The model under review builds one solid part; all positions refer to its coordinate system, in mm. A direction names the side the tool comes from. Round coordinates to 2 decimals unless told otherwise and drop trailing zeros. Write each loop counter-clockwise with the first axis right and the second up, starting at its lowest first coordinate (ties: lowest second). Pieces come first, ordered by that corner, then holes. Notation, with made-up numbers: (6.5, -39) - (44.5, -39) arc R33 cw to (44.5, -3) - close; hole circle Ø2 at (3, 59.5). An arc over 180 degrees is marked (long way). Return JSON: item names as keys, results as strings.
from build123d import *

# Parameters (mm, degrees)
SKETCH1_W                   = 224.46234
SKETCH1_H                   = 149.606
BOSS_EXTRUDE1_DEPTH         = 2.54
SKETCH2_W                   = 44.45
SKETCH2_H                   = 87.5411
CUT_EXTRUDE1_DEPTH          = 135.899132423
F_1_4_CLEARANCE_HOLE1_D     = 6.5278
F_1_4_CLEARANCE_HOLE1_DEPTH = 9.398
F_1_4_CLEARANCE_HOLE1_TIP   = 1.961148974
SKETCH6_W                   = 25.4
SKETCH6_H                   = 2.54
CUT_EXTRUDE2_DEPTH          = 135.899132423
LPATTERN1_COUNT             = 4
LPATTERN1_PITCH             = 50.8
SKETCH7_W                   = 2.54
SKETCH7_H                   = 21.59
CUT_EXTRUDE3_DEPTH          = 135.899132423
LPATTERN2_COUNT             = 3
LPATTERN2_PITCH             = 43.18
SKETCH8_R                   = 9.525
CUT_EXTRUDE4_DEPTH          = 135.899132423
SKETCH9_R                   = 15.875
SKETCH9_W                   = 44.7802
SKETCH9_H                   = 69.85
CUT_EXTRUDE5_DEPTH          = 135.899132423
FILLET2_R                   = 12.7
SKETCH25_W                  = 12.7
SKETCH25_H                  = 147.066
BOSS_EXTRUDE5_DEPTH         = 2.54
SKETCH16_W                  = 2.54
SKETCH16_H                  = 25.4
BOSS_EXTRUDE2_DEPTH         = 2.54
SKETCH23_W                  = 44.45
SKETCH23_H                  = 87.5411
BOSS_EXTRUDE3_DEPTH         = 2.54
SKETCH24_W                  = 33.3375
SKETCH24_H                  = 149.606
BOSS_EXTRUDE4_DEPTH         = 2.54
LPATTERN3_COUNT             = 3
LPATTERN3_PITCH             = 50.8
LPATTERN3_COUNT_DIR2        = 2
LPATTERN3_PITCH_DIR2        = 273.03984
SKETCH18_W                  = 275.57984
SKETCH18_H                  = 5.334
CUT_EXTRUDE7_DEPTH          = 169.417839014
M3_CLEARANCE_HOLE1_D        = 3.2
M3_CLEARANCE_HOLE1_DEPTH    = 9.398
M3_CLEARANCE_HOLE1_TIP      = 0.96137699
SKETCH27_W                  = 73.9775
SKETCH27_H                  = 58.7375
CUT_EXTRUDE9_DEPTH          = 2.54
CUT_EXTRUDE10_DEPTH         = 2.54
SKETCH29_W                  = 25.4
SKETCH29_H                  = 2.54
CUT_EXTRUDE11_DEPTH         = 166.946131435
LPATTERN4_COUNT             = 5
LPATTERN4_PITCH             = 50.8


with BuildPart() as part:
    # Sketch1 → Boss-Extrude1 (new body)
    with BuildSketch(Plane(origin=(0, 0, 0), x_dir=(0, 0, -1), z_dir=(1, 0, 0))):
        Rectangle(SKETCH1_W, SKETCH1_H)
    extrude(amount=BOSS_EXTRUDE1_DEPTH)

    # Sketch2 → Cut-Extrude1 (cut, through all)
    with BuildSketch(Plane(origin=(2.54, 0, 0), x_dir=(0, 0, -1), z_dir=(1, 0, 0))):
        with Locations((90.00617, 31.03245)):
            Rectangle(SKETCH2_W, SKETCH2_H)
    extrude(amount=-CUT_EXTRUDE1_DEPTH, mode=Mode.SUBTRACT)

    # 1/4 Clearance Hole1
    with Locations(Plane(origin=(2.54, 0, 0), x_dir=(0, 0, -1), z_dir=(1, 0, 0))):
        with Locations((-81.69783, -64.77), (-62.01283, -64.77), (102.09657, -64.77), (82.41157, -64.77)):
            Hole(F_1_4_CLEARANCE_HOLE1_D / 2, depth=F_1_4_CLEARANCE_HOLE1_DEPTH)
            with Locations((0, 0, -(F_1_4_CLEARANCE_HOLE1_DEPTH + F_1_4_CLEARANCE_HOLE1_TIP / 2))):  # 118° drill point
                Cone(0, F_1_4_CLEARANCE_HOLE1_D / 2, F_1_4_CLEARANCE_HOLE1_TIP, mode=Mode.SUBTRACT)

    # Sketch6 → Cut-Extrude2 (cut, through all)
    with BuildSketch(Plane(origin=(2.54, 0, 0), x_dir=(0, 0, -1), z_dir=(1, 0, 0))):
        with Locations((39.84117, 73.533)):
            Rectangle(SKETCH6_W, SKETCH6_H)
    cut_extrude2 = extrude(amount=-CUT_EXTRUDE2_DEPTH, mode=Mode.SUBTRACT)

    # LPattern1: Cut-Extrude2 ×4
    with Locations(*[(0, 0, i * LPATTERN1_PITCH) for i in range(1, LPATTERN1_COUNT)]):
        add(cut_extrude2, mode=Mode.SUBTRACT)

    # Sketch7 → Cut-Extrude3 (cut, through all)
    with BuildSketch(Plane(origin=(2.54, 0, 0), x_dir=(0, 0, -1), z_dir=(1, 0, 0))):
        with Locations((66.51117, 53.213)):
            Rectangle(SKETCH7_W, SKETCH7_H)
    cut_extrude3 = extrude(amount=-CUT_EXTRUDE3_DEPTH, mode=Mode.SUBTRACT)

    # LPattern2: Cut-Extrude3 ×3
    with Locations(*[(0, -i * LPATTERN2_PITCH, 0) for i in range(1, LPATTERN2_COUNT)]):
        add(cut_extrude3, mode=Mode.SUBTRACT)

    # Sketch8 → Cut-Extrude4 (cut, through all)
    with BuildSketch(Plane(origin=(2.54, 0, 0), x_dir=(0, 0, -1), z_dir=(1, 0, 0))):
        with Locations((92.22867, -39.7370046)):
            Circle(SKETCH8_R)
        with Locations((-71.82993, -39.7370046)):
            Circle(SKETCH8_R)
    extrude(amount=-CUT_EXTRUDE4_DEPTH, mode=Mode.SUBTRACT)

    # Sketch9 → Cut-Extrude5 (cut, through all)
    with BuildSketch(Plane(origin=(2.54, 0, 0), x_dir=(0, 0, -1), z_dir=(1, 0, 0))):
        with Locations((-67.78625, 31.7373)):
            Circle(SKETCH9_R)
        with Locations((3.84937, -39.878)):
            Rectangle(SKETCH9_W, SKETCH9_H)
    extrude(amount=-CUT_EXTRUDE5_DEPTH, mode=Mode.SUBTRACT)

    # Fillet2
    fillet2_edges = [part.edges().sort_by_distance(p)[0] for p in [
        (1.27, -74.803, 18.54073),
        (1.27, -4.953, 18.54073),
        (1.27, -4.953, -26.23947),
        (1.27, -74.803, -26.23947),
    ]]
    fillet(fillet2_edges, radius=FILLET2_R)

    # Sketch25 → Boss-Extrude5 (add)
    with BuildSketch(Plane(origin=(2.54, 0, 0), x_dir=(0, 0, -1), z_dir=(1, 0, 0))):
        with Locations((-118.58117, -1.27)):
            Rectangle(SKETCH25_W, SKETCH25_H)
    extrude(amount=-BOSS_EXTRUDE5_DEPTH)

    # Sketch16 → Boss-Extrude2 (add)
    with BuildSketch(Plane(origin=(2.54, 0, 0), x_dir=(0, 0, -1), z_dir=(1, 0, 0))):
        with Locations((-126.20117, 34.163)):
            Rectangle(SKETCH16_W, SKETCH16_H)
    boss_extrude2 = extrude(amount=-BOSS_EXTRUDE2_DEPTH)

    # Sketch23 → Boss-Extrude3 (add)
    with BuildSketch(Plane(origin=(2.54, 0, 0), x_dir=(0, 0, -1), z_dir=(1, 0, 0))):
        with Locations((90.00617, 31.03245)):
            Rectangle(SKETCH23_W, SKETCH23_H)
    extrude(amount=-BOSS_EXTRUDE3_DEPTH)

    # Sketch24 → Boss-Extrude4 (add)
    with BuildSketch(Plane(origin=(2.54, 0, 0), x_dir=(0, 0, -1), z_dir=(1, 0, 0))):
        with Locations((128.89992, 0)):
            Rectangle(SKETCH24_W, SKETCH24_H)
    extrude(amount=-BOSS_EXTRUDE4_DEPTH)

    # LPattern3: Boss-Extrude2 3 × 2
    with Locations(*[(0, -i * LPATTERN3_PITCH, -j * LPATTERN3_PITCH_DIR2) for i in range(LPATTERN3_COUNT) for j in range(LPATTERN3_COUNT_DIR2) if (i, j) != (0, 0)]):
        add(boss_extrude2)

    # Sketch18 → Cut-Extrude7 (cut, through all)
    with BuildSketch(Plane(origin=(2.54, 0, 0), x_dir=(0, 0, -1), z_dir=(1, 0, 0))):
        with Locations((10.31875, -77.47)):
            Rectangle(SKETCH18_W, SKETCH18_H)
    extrude(amount=-CUT_EXTRUDE7_DEPTH, mode=Mode.SUBTRACT)

    # M3 Clearance Hole1
    with Locations(Plane(origin=(2.54, 0, 0), x_dir=(0, 0, -1), z_dir=(1, 0, 0))):
        with Locations((-115.40617, 62.738), (55.71617, 62.738)):
            Hole(M3_CLEARANCE_HOLE1_D / 2, depth=M3_CLEARANCE_HOLE1_DEPTH)
            with Locations((0, 0, -(M3_CLEARANCE_HOLE1_DEPTH + M3_CLEARANCE_HOLE1_TIP / 2))):  # 118° drill point
                Cone(0, M3_CLEARANCE_HOLE1_D / 2, M3_CLEARANCE_HOLE1_TIP, mode=Mode.SUBTRACT)

    # Sketch27 → Cut-Extrude9 (cut)
    with BuildSketch(Plane(origin=(2.54, 0, 0), x_dir=(0, 0, -1), z_dir=(1, 0, 0))):
        with Locations((111.11992, 45.43425)):
            Rectangle(SKETCH27_W, SKETCH27_H)
    extrude(amount=-CUT_EXTRUDE9_DEPTH, mode=Mode.SUBTRACT)

    # Sketch28 → Cut-Extrude10 (cut)
    with BuildSketch(Plane.ZY):
        with BuildLine():
            Line((-111.27867, -31.1010046), (-111.27867, -39.7370046))
            Line((-111.27867, -39.7370046), (-73.17867, -39.7370046))
            Line((-73.17867, -39.7370046), (-73.17867, -31.1010046))
            ThreePointArc((-73.17867, -31.1010046), (-92.22867, -12.0510046), (-111.27867, -31.1010046))
        make_face()
        with BuildLine():
            Line((52.77993, -31.1010046), (52.77993, -39.7370046))
            Line((52.77993, -39.7370046), (90.87993, -39.7370046))
            Line((90.87993, -39.7370046), (90.87993, -31.1010046))
            ThreePointArc((90.87993, -31.1010046), (71.82993, -12.0510046), (52.77993, -31.1010046))
        make_face()
    extrude(amount=-CUT_EXTRUDE10_DEPTH, mode=Mode.SUBTRACT)

    # Sketch29 → Cut-Extrude11 (cut, through all)
    with BuildSketch(Plane(origin=(2.54, 0, 0), x_dir=(0, 0, -1), z_dir=(1, 0, 0))):
        with Locations((135.40867, 14.7955)):
            Rectangle(SKETCH29_W, SKETCH29_H)
    cut_extrude11 = extrude(amount=-CUT_EXTRUDE11_DEPTH, mode=Mode.SUBTRACT)

    # LPattern4: Cut-Extrude11 ×5
    with Locations(*[(0, 0, i * LPATTERN4_PITCH) for i in range(1, LPATTERN4_COUNT)]):
        add(cut_extrude11, mode=Mode.SUBTRACT)


solid = part.part
(1) Clearance check with flat-ended pins moving along their axes: pin 1 Ø1.3 at (x, z) = (1, -35) entering from +Y; pin 2 Ø0.8 at (x, z) = (1.5, -30) entering from -Y; pin 3 Ø1.3 at (x, y) = (2, 34) entering from -Z. State where each tip first meets the part, or that it passes through.
Filled in:
{"pin 1": "stops at y = 72.26", "pin 2": "stops at y = -71.5", "pin 3": "stops at z = -74.13"}
(2) Mouldability with a two-part tool opening along Y and no side actions: class faces 4 (the cylindrical face through (1.252, -8.772, -22.618)), 5 (the flat face through (0, 1, -8)), 6 (the cylindrical face through (1.252, -12.056, 72.249)) as released by +Y, released by -Y, zero draft, split by the parting line, or undercut.
Filled in:
{"face 4": "released by -Y", "face 5": "zero draft", "face 6": "undercut"}
(3) For faces 1 (the cylindrical face through (1.29, -49.26, 72.04)), 2 (the cylindrical face through (1.25, -71.18, 22.36)), 3 (the flat face through (2.54, 1, -8)), list the 3-axis set-ups (+Z, -Z, +X, -X, +Y, -Y) from which the entire face can be reached by the end or side of a thin tool; tool diameter is ignored.
Filled in:
{"face 1": "+X, -X", "face 2": "+X, -X, -Y", "face 3": "+Z, -Z, +X, +Y, -Y"}
(4) Add section A-A (y = -52). Write out the cut boundary in (x, z), plus the area to 3 significant figures.
Filled in:
{"outline": "(0, -145.57) - (2.54, -145.57) - (2.54, -26.24) - (0, -26.24) - close; (0, 18.54) - (2.54, 18.54) - (2.54, 124.93) - (0, 124.93) - close", "area": "573 mm2"}
(5) Wall thickness on line 1 (Y direction, x = 0.1, z = -67); line 2 (Z direction, x = 2.35, y = 16); line 3 (Z direction, x = 2.35, y = 7): over which ranges is each line inside the solid? List them lowest first.
Filled in:
{"line 1": "y = -74.8 to -43.94, -22.35 to -0.76, 20.83 to 42.42, 64.01 to 74.8", "line 2": "z = -122.71 to -97.31, -71.91 to -67.78, -65.24 to -46.51, -21.11 to 4.29, 29.69 to 55.09, 80.49 to 124.93", "line 3": "z = -145.57 to -67.78, -65.24 to 124.93"}
(6) Add section B-B (z = 9). Write out the cut boundary in (x, y).
Filled in:
{"outline": "(0, -5.35) - (2.54, -5.35) - (2.54, 13.53) - (0, 13.53) - close; (0, 16.07) - (2.54, 16.07) - (2.54, 72.26) - (0, 72.26) - close"}
